Read the model definition and answer for the solid it produces. Units are mm, in the model's axes. A direction names the side the tool comes from. Coordinates: 2 decimals unless noted, no trailing zeros. Order: outer loops, then holes, each group sorted by start corner. A loop starts at its lowest first (then second) coordinate and runs counter-clockwise, first axis right, second up. Notation, with made-up numbers: (89.25, 88.25) -> (98.25, 88.25) arc R25 ccw to (98.25, 127.25) -> close; hole circle Ø5 at (3, 73). An arc over 180 degrees is marked (long way). Answer in a Markdown table with one row per item.
from build123d import *

# Parameters (mm, degrees)
SKETCH1_R           = 10
BOSS_EXTRUDE1_DEPTH = 3
SKETCH3_R           = 8
SKETCH3_R_2         = 6.5
CUT_EXTRUDE1_DEPTH  = 1
SKETCH4_R           = 1.25
CUT_EXTRUDE2_DEPTH  = 15.456832295


with BuildPart() as part:
    # Sketch1 → Boss-Extrude1 (new body)
    with BuildSketch(Plane(origin=(0, 0, 0), x_dir=(1, 0, 0), z_dir=(0, 1, 0))):
        with Locations(Location((0, 0, 0), (0, 0, 270))):
            Circle(SKETCH1_R)
    extrude(amount=BOSS_EXTRUDE1_DEPTH)

    # Sketch3 → Cut-Extrude1 (cut)
    with BuildSketch(Plane(origin=(0, 3, 0), x_dir=(1, 0, 0), z_dir=(0, 1, 0))):
        with Locations(Location((0, 0, 0), (0, 0, 270))):
            Circle(SKETCH3_R)
        with Locations(Location((0, 0, 0), (0, 0, 270))):
            Circle(SKETCH3_R_2, mode=Mode.SUBTRACT)
    extrude(amount=-CUT_EXTRUDE1_DEPTH, mode=Mode.SUBTRACT)

    # Sketch4 → Cut-Extrude2 (cut, through all)
    with BuildSketch(Plane(origin=(0, 0, 0), x_dir=(1, 0, 0), z_dir=(0, 1, 0))):
        with Locations(Location((4.25, 0, 0), (0, 0, 270))):
            Circle(SKETCH4_R)
        with Locations(Location((-4.25, 0, 0), (0, 0, 90))):
            Circle(SKETCH4_R)
    extrude(amount=CUT_EXTRUDE2_DEPTH, mode=Mode.SUBTRACT)


solid = part.part
Q1. For faces 4 (the face through (-3, 1, 0)), 5 (the face through (-7.81, 2.51, -1.73)), determine the directions among +Z, -Z, +X, -X, +Y, -Y from which every point of the face is accessible in a straight line to the end or side of a thin tool.
Outcome:
| item | result |
|---|---|
| face 4 | +Y, -Y |
| face 5 | +Y |
Q2. Consider line 1 (X direction, y = 2.3, z = 0); line 2 (X direction, y = 0.8, z = 0); line 3 (Z direction, x = -2, y = 2.85). Determine where each line is inside the solid, lowest interval first.
Outcome:
| item | result |
|---|---|
| line 1 | -10 to -8, -6.5 to -5.5, -3 to 3, 5.5 to 6.5, 8 to 10 |
| line 2 | -10 to -5.5, -3 to 3, 5.5 to 10 |
| line 3 | -9.8 to -7.75, -6.18 to 6.18, 7.75 to 9.8 |
Q3. The part is cut by section D-D (x = -4.25). Write down the section's boundary in (y, z), then the cut area to 3 significant figures.
Outcome:
| item | result |
|---|---|
| outline | (0, -9.05) -> (3, -9.05) -> (3, -6.78) -> (2, -6.78) -> (2, -4.92) -> (3, -4.92) -> (3, -1.25) -> (0, -1.25) -> close; (0, 1.25) -> (3, 1.25) -> (3, 4.92) -> (2, 4.92) -> (2, 6.78) -> (3, 6.78) -> (3, 9.05) -> (0, 9.05) -> close |
| area | 43.1 mm² |
Q4. For a pull along X with two mould halves and no side action, classify faces 1 (the face through (0, 3, 0)), 2 (the face through (-9.76, 1.48, -2.17)), 3 (the face through (7, 2, 0)) as pulls with the +X half, pulls with the -X half, needs draft (parallel to the pull), parting line crosses it, or undercut.
Outcome:
| item | result |
|---|---|
| face 1 | needs draft |
| face 2 | parting line crosses it |
| face 3 | undercut |
Q5. The part is cut by section A-A (y = 2.25). Write down the section's boundary in (x, z), then the cut area to 3 significant figures.
Outcome:
| item | result |
|---|---|
| outline | circle Ø20 at (0, 0); circle Ø13 at (0, 0); hole circle Ø16 at (0, 0); hole circle Ø2.5 at (-4.25, 0); hole circle Ø2.5 at (4.25, 0) |
| area | 236 mm² |
Q6. The part is cut by section B-B (z = 0). Write down the section's boundary in (x, y).
Outcome:
| item | result |
|---|---|
| outline | (-10, 0) -> (-5.5, 0) -> (-5.5, 3) -> (-6.5, 3) -> (-6.5, 2) -> (-8, 2) -> (-8, 3) -> (-10, 3) -> close; (-3, 0) -> (3, 0) -> (3, 3) -> (-3, 3) -> close; (5.5, 0) -> (10, 0) -> (10, 3) -> (8, 3) -> (8, 2) -> (6.5, 2) -> (6.5, 3) -> (5.5, 3) -> close |
Q7. Given pin 1 (1.5 mm diameter, centred on x = 4.25, z = 0, fed in from -Y), flat-ended and moving along its own axis, determine where the tip first touches the part or whether it passes through.
Outcome:
| item | result |
|---|---|
| pin 1 | through |
Q8. The part is cut by section C-C (x = 0). Write down the section's boundary in (y, z), then the cut area to 3 significant figures.
Outcome:
| item | result |
|---|---|
| outline | (0, -10) -> (3, -10) -> (3, -8) -> (2, -8) -> (2, -6.5) -> (3, -6.5) -> (3, 6.5) -> (2, 6.5) -> (2, 8) -> (3, 8) -> (3, 10) -> (0, 10) -> close |
| area | 57.0 mm² |
